The model under review builds one solid part; all positions refer to its coordinate system, in mm. A direction names the side the tool comes from. Round coordinates to 2 decimals unless told otherwise and drop trailing zeros. Order: outer loops, then holes, each group sorted by start corner. A loop starts at its lowest first (then second) coordinate and runs counter-clockwise, first axis right, second up. Notation, with made-up numbers: (55.5, 25.5) -> (103.5, 25.5) arc R34 ccw to (103.5, 57.5) -> close; hole circle Ø10 at (89.5, 54). An arc over 180 degrees is marked (long way). Put each result on its own line as item: value. Start each with the question number.
from build123d import *

# Parameters (mm, degrees)
SKETCH1_R           = 22
BOSS_EXTRUDE1_DEPTH = 10
SKETCH2_R           = 12.5
BOSS_EXTRUDE2_DEPTH = 6.1
SKETCH3_R           = 22
SKETCH3_R_2         = 18.85
CUT_EXTRUDE2_DEPTH  = 8
SKETCH5_R           = 22
BOSS_EXTRUDE3_DEPTH = 2
SKETCH6_R           = 2.25
CUT_EXTRUDE3_DEPTH  = 28


with BuildPart() as part:
    # Sketch1 → Boss-Extrude1 (new body)
    with BuildSketch(Plane(origin=(0, 0, 0), x_dir=(1, 0, 0), z_dir=(0, 1, 0))):
        Circle(SKETCH1_R)
    extrude(amount=BOSS_EXTRUDE1_DEPTH)

    # Sketch2 → Boss-Extrude2 (add)
    with BuildSketch(Plane(origin=(0, 10, 0), x_dir=(1, 0, 0), z_dir=(0, 1, 0))):
        Circle(SKETCH2_R)
    extrude(amount=BOSS_EXTRUDE2_DEPTH)

    # Sketch3 → Cut-Extrude2 (cut)
    with BuildSketch(Plane.XZ):
        Circle(SKETCH3_R)
        Circle(SKETCH3_R_2, mode=Mode.SUBTRACT)
    extrude(amount=-CUT_EXTRUDE2_DEPTH, mode=Mode.SUBTRACT)

    # Sketch5 → Boss-Extrude3 (add)
    with BuildSketch(Plane.XZ):
        Circle(SKETCH5_R)
    extrude(amount=BOSS_EXTRUDE3_DEPTH)

    # Sketch6 → Cut-Extrude3 (cut)
    with BuildSketch(Plane.XZ.offset(2)):
        Circle(SKETCH6_R)
    extrude(amount=-CUT_EXTRUDE3_DEPTH, mode=Mode.SUBTRACT)


solid = part.part
Q1. Wall thickness on probe 1 along Y at (x, z) = (-10.5, 17); probe 2 along Z at (x, y) = (0, 4.75); probe 3 along Y at (x, z) = (8, 11): over which ranges is each line inside the solid? List them lowest first. Write a range as [from, to].
Q2. Clearance check with flat-ended pins moving along their axes: pin 1 Ø4 at (x, z) = (5.5, -16) entering from +Y; pin 2 Ø10 at (x, y) = (15, 4) entering from -Z; pin 3 Ø2 at (x, y) = (-2.5, 13.5) entering from +Z. State where each tip first meets the part, or that it passes through.
Q3. Draft analysis for pull direction Y (two halves, no side actions). For faces 4 (the face through (-4.1, 3.9, -18.4)), 5 (the face through (-4.769, 8.986, 21.477)), 6 (the face through (18, 8, 7)), 7 (the face through (9, 10, 9)), state which applies: +Y half, -Y half, draft (parallel to the pull), parting line (faces both ways), or undercut.
Q4. Take a section at B-B on x = 0. Give the boundary of the cut face in (y, z).
Q5. Take a section at C-C on y = 9. Give the boundary of the cut face in (x, z).
Q6. Take a section at A-A on z = 0. Give the boundary of the cut face in (x, y), and give its area (3 significant figures).
Q7. For faces 1 (the face through (18, 0, 7)), 2 (the face through (0, 16.1, 3)), 3 (the face through (11.923, 13.007, -3.755)), list the 3-axis set-ups (+Z, -Z, +X, -X, +Y, -Y) from which the entire face can be reached by the end or side of a thin tool; tool diameter is ignored.
Q8. Take a section at D-D on z = 9.5. Give the boundary of the cut face in (x, y).
Calculated:
1. probe 1: y = [-2, 0], [8, 10]
1. probe 2: z = [-18.85, -2.25], [2.25, 18.85]
1. probe 3: y = [-2, 10]
2. pin 1: stops at y = 10
2. pin 2: stops at z = -18.44
2. pin 3: stops at z = 12.41
3. face 4: undercut
3. face 5: draft
3. face 6: undercut
3. face 7: +Y half
4. outline: (-2, -22) -> (0, -22) -> (0, -18.85) -> (8, -18.85) -> (8, -22) -> (10, -22) -> (10, -12.5) -> (16.1, -12.5) -> (16.1, -2.25) -> (-2, -2.25) -> close; (-2, 2.25) -> (16.1, 2.25) -> (16.1, 12.5) -> (10, 12.5) -> (10, 22) -> (8, 22) -> (8, 18.85) -> (0, 18.85) -> (0, 22) -> (-2, 22) -> close
5. outline: circle Ø44 at (0, 0); hole circle Ø4.5 at (0, 0)
6. outline: (-22, -2) -> (-2.25, -2) -> (-2.25, 16.1) -> (-12.5, 16.1) -> (-12.5, 10) -> (-22, 10) -> (-22, 8) -> (-18.85, 8) -> (-18.85, 0) -> (-22, 0) -> close; (2.25, -2) -> (22, -2) -> (22, 0) -> (18.85, 0) -> (18.85, 8) -> (22, 8) -> (22, 10) -> (12.5, 10) -> (12.5, 16.1) -> (2.25, 16.1) -> close
6. area: 549 mm²
7. face 1: none
7. face 2: +Z, -Z, +X, -X, +Y
7. face 3: +Y
8. outline: (-19.84, -2) -> (19.84, -2) -> (19.84, 0) -> (16.28, 0) -> (16.28, 8) -> (19.84, 8) -> (19.84, 10) -> (8.12, 10) -> (8.12, 16.1) -> (-8.12, 16.1) -> (-8.12, 10) -> (-19.84, 10) -> (-19.84, 8) -> (-16.28, 8) -> (-16.28, 0) -> (-19.84, 0) -> close
